Geometry check sheet. Reference: the model listing, model coordinates, mm. Face numbers are marked on the shaded views. A direction names the side the tool comes from. Coordinates: 2 decimals unless noted, no trailing zeros. Write each loop counter-clockwise with the first axis right and the second up, starting at its lowest first coordinate (ties: lowest second). Pieces come first, ordered by that corner, then holes. Notation, with made-up numbers: (9.25, 76.25) -> (36.25, 76.25) arc R20 ccw to (36.25, 84.25) -> close; hole circle Ø9 at (37.25, 75.25). An arc over 180 degrees is marked (long way). Answer in a Markdown table with one row per item. Add a question column.
1. Mould release check, pull along Z, two halves, no side actions. Record for the marked faces 1, 2 and 3: pulls with the +Z half, pulls with the -Z half, needs draft (parallel to the pull), parting line crosses it, or undercut.
2. Cross-section at B-B on z = 11.5. Record the cut outline in (x, y) (3 decimals).
3. Cross-section at A-A on y = 68. Record the cut outline in (x, z), and give its area (3 significant figures).
4. Set-up check for the marked faces 4, 5, 6 and 7: record each of +Z, -Z, +X, -X, +Y, -Y from which the full face is reachable in a straight line by a thin tool's end or side.
5. Cross-section at D-D on y = 50.8. Record the cut outline in (x, z), and give its area (3 significant figures).
6. Depth check by flat-ended pin: P1, Ø22, axis at y = 38.5, z = 2.5, coming from the +X side; P2, Ø19, axis at y = 51, z = -13.5, coming from the -X side; P3, Ø19, axis at y = 51, z = -9, coming from the +X side; P4, Ø19, axis at x = 36.5, z = -14.5, coming from the -Y side. Enter the tip coordinate at first touch or a pass-through.
7. Scan lines: L1, parallel to Z at x = 63.5, y = 59; L2, parallel to X at y = 29.5, z = 4.5; L3, parallel to X at y = 50.8, z = 15.75. Record each from-to range of solid material in increasing order. Write a range as from..to.
8. Cross-section at C-C on x = -7.5. Record the cut outline in (y, z).
```python
from build123d import *

# Parameters (mm, degrees)
F0_W          = 101.6
F0_H          = 38.089089331
F1_DEPTH      = 101.6
F2_DEPTH      = 114.3
F2_DEPTH_BACK = 12.7
F3_W          = 25.4
F3_H          = 20.1185690239
F4_DEPTH      = 114.301
F6_D          = 19.05
F6_DEPTH      = 19.05
F6_TIP        = 5.7231973962


with BuildPart() as f1:
    # F0 (on Front) → F1 (new body)
    with BuildSketch(Plane.XZ):
        with Locations((11.9261237085, -10.133718954)):
            Rectangle(F0_W, F0_H)
    extrude(amount=-F1_DEPTH)

    # F0 (on Front) → F2 (join, two sides)
    with BuildSketch(Plane.XZ) as f2_sk:
        Polygon((75.4261237085, 27.9608257115), (-51.5738762915, 27.9608257115), (-51.5738762915, 8.9108257115), (-38.8738762915, 8.9108257115), (62.7261237085, 8.9108257115), (75.4261237085, 8.9108257115), align=None)
        Polygon((62.7261237085, -29.1782636195), (-38.8738762915, -29.1782636195), (-51.5738762915, -29.1782636195), (-51.5738762915, -48.2282636195), (75.4261237085, -48.2282636195), (75.4261237085, -29.1782636195), align=None)
    extrude(amount=-F2_DEPTH)
    extrude(f2_sk.sketch, amount=F2_DEPTH_BACK)

    # F3 (on Front) → F4 (cut, through all)
    with BuildSketch(Plane.XZ):
        with Locations((12.7, -2.1666153334)):
            Rectangle(F3_W, F3_H)
    extrude(amount=-F4_DEPTH, mode=Mode.SUBTRACT)

    # F6
    with Locations(Plane.XY.offset(27.9608257115)):
        with Locations((11.9261237085, 50.8)):
            Hole(F6_D / 2, depth=F6_DEPTH)
            with Locations((0, 0, -(F6_DEPTH + F6_TIP / 2))):  # 118° drill point
                Cone(0, F6_D / 2, F6_TIP, mode=Mode.SUBTRACT)


solid = f1.part
```
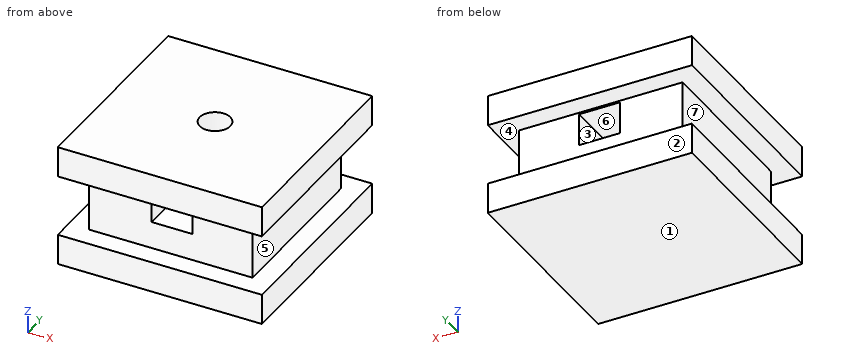
Results found:
| question | item | result |
|---|---|---|
| 1 | face 1 | pulls with the -Z half |
| 1 | face 2 | needs draft |
| 1 | face 3 | undercut |
| 2 | outline | (-51.574, -12.7) -> (75.426, -12.7) -> (75.426, 114.3) -> (-51.574, 114.3) -> close; hole circle Ø19.05 at (11.926, 50.8) |
| 3 | outline | (-51.57, -48.23) -> (75.43, -48.23) -> (75.43, -29.18) -> (62.73, -29.18) -> (62.73, 8.91) -> (75.43, 8.91) -> (75.43, 27.96) -> (-51.57, 27.96) -> (-51.57, 8.91) -> (-38.87, 8.91) -> (-38.87, -29.18) -> (-51.57, -29.18) -> close; hole (0, -12.23) -> (25.4, -12.23) -> (25.4, 7.89) -> (0, 7.89) -> close |
| 3 | area | 8,200 mm^2 |
| 4 | face 4 | none |
| 4 | face 5 | +X, +Y, -Y |
| 4 | face 6 | +Y, -Y |
| 4 | face 7 | -X, +Y, -Y |
| 5 | outline | (-51.57, -48.23) -> (75.43, -48.23) -> (75.43, -29.18) -> (62.73, -29.18) -> (62.73, 8.91) -> (75.43, 8.91) -> (75.43, 27.96) -> (21.45, 27.96) -> (21.45, 8.91) -> (19.76, 7.89) -> (25.4, 7.89) -> (25.4, -12.23) -> (0, -12.23) -> (0, 7.89) -> (4.1, 7.89) -> (2.4, 8.91) -> (2.4, 27.96) -> (-51.57, 27.96) -> (-51.57, 8.91) -> (-38.87, 8.91) -> (-38.87, -29.18) -> (-51.57, -29.18) -> close |
| 5 | area | 7,820 mm^2 |
| 6 | P1 | stops at x = 75.43 |
| 6 | P2 | stops at x = -38.87 |
| 6 | P3 | stops at x = 62.73 |
| 6 | P4 | stops at y = 0 |
| 7 | L1 | z = -48.23..-29.18, 8.91..27.96 |
| 7 | L2 | x = -38.87..0, 25.4..62.73 |
| 7 | L3 | x = -51.57..2.4, 21.45..75.43 |
| 8 | outline | (-12.7, -48.23) -> (114.3, -48.23) -> (114.3, -29.18) -> (101.6, -29.18) -> (101.6, 8.91) -> (114.3, 8.91) -> (114.3, 27.96) -> (-12.7, 27.96) -> (-12.7, 8.91) -> (0, 8.91) -> (0, -29.18) -> (-12.7, -29.18) -> close |
